For this review, take the finished solid that the model builds, in its own axes (mm). A direction names the side the tool comes from. Give positions to 0.01 mm unless a question says otherwise; leave off trailing zeros. Write each loop counter-clockwise with the first axis right and the second up, starting at its lowest first coordinate (ties: lowest second). Pieces come first, ordered by that corner, then holes. Notation, with made-up numbers: M 52,60.25 L 71,60.25 A16 cw 71,68.25 Z; hole C 66,1.5 d9. An arc over 180 degrees is marked long. Write item = value, one per line.
```python
from build123d import *

# Parameters (mm, degrees)
FILLET_1_R = 0.5


with BuildPart() as part:
    # Эскиз1 → Повернуть1 (revolve)
    with BuildSketch(Plane(origin=(0, 0, 0), x_dir=(1, 0, 0), z_dir=(0, 1, 0)), mode=Mode.PRIVATE) as revolve_1_sk:
        Polygon((-20.31661762, 2), (-20.31661762, 3), (-19.31661762, 3), (-19.31661762, 4.5), (-9.31661762, 4.5), (-7.005272431, 3.180480624), (1.994727569, 3.180480624), (2.462581397, 4), (5.68338238, 4), (5.68338238, 2), align=None)
    revolve(revolve_1_sk.sketch.rotate(Axis((-48.681122779, 0, 0), (1, 0, 0)), 180), axis=Axis((-48.681122779, 0, 0), (1, 0, 0)))

    # Скругление1
    fillet_1_edges = [part.edges().sort_by_distance(p)[0] for p in [
        (-19.31661762, 0, -4.5),
        (-9.31661762, 0, -4.5),
        (-7.005272431, 0, -3.180480624),
        (1.994727569, 0, -3.180480624),
        (2.462581397, 0, -4),
        (5.68338238, 0, -4),
    ]]
    fillet(fillet_1_edges, radius=FILLET_1_R)


solid = part.part
```
1. We need section A-A, the plane x = 0.5. Write out the cut boundary in (y, z).
Responses:
outline = C 0,0 d6.36; hole C 0,0 d4
2. Machinability: for faces 1 (the face through (3.985, 3.905, -0.867)), 2 (the face through (5.683, 2, 2)), 3 (the face through (-19.81, -0.9, 2.86)), which of the approach directions +Z, -Z, +X, -X, +Y, -Y give a long, thin tool a straight path to every point of the face, cutting with its end or side? Answer none if there is none.
Responses:
face_1 = +X
face_2 = +Z, -Z, +X, +Y, -Y
face_3 = -X
3. We need section B-B, the plane x = -12. Write out the cut boundary in (y, z), then the cut area to 3 significant figures.
Responses:
outline = C 0,0 d9; hole C 0,0 d4
area = 51.1 mm2
4. For line 1 along Y through (x, z) = (-9.75, 0); line 2 along Y through (x, z) = (-0.5, 0); line 3 along Z through (x, y) = (-14.25, -1), list the stretches that pass through material, from the lowest coordinate up. Write a range as from..to.
Responses:
line_1 = -4.5..-2, 2..4.5
line_2 = -3.18..-2, 2..3.18
line_3 = -4.39..-1.73, 1.73..4.39
5. Insertion check: P1, Ø1.5, axis at x = -11, z = -1.5, coming from the +Y side; P2, Ø5, axis at x = -14, y = 3, coming from the -Z side; P3, Ø4, axis at y = -1.5, z = 0, coming from the +X side; P4, Ø3, axis at x = -7, y = 2.5, coming from the +Z side. Each pin has a flat end and moves straight along its axis. Give the tip position at first contact, or say it passes through.
Responses:
P1 = 4.44
P2 = -4.47
P3 = 5.68
P4 = 3.52
6. The part is to be moulded in two halves that separate along X. For faces 4 (the face through (-20.317, 2, -1)), 5 (the face through (-14.07, 1.72, 4.16)), 6 (the face through (-2.524, -0.955, 3.034)), say which applies: +X half, -X half, draft (parallel to the pull), parting line (faces both ways), or undercut.
Responses:
face_4 = -X half
face_5 = draft
face_6 = undercut
